Answer from the drawing. Dimensions are ordinates in mm from the lowest x, y and z of the part. A direction names the side the tool comes from. Coordinates: 2 decimals unless noted, no trailing zeros. Write each loop counter-clockwise with the first axis right and the second up, starting at its lowest first coordinate (ties: lowest second). Pieces come first, ordered by that corner, then holes.
(1) The part is cut by section B-B on z = 7.5. Determine the outline of the cut face in (x, y), plus the area to 3 significant figures.
(2) The part is cut by section D-D on x = 13.5. Determine the outline of the cut face in (y, z).
(3) The part is cut by section A-A on x = 7.5. Determine the outline of the cut face in (y, z).
(4) For a pull along Z with two mould halves and no side action, classify the marked faces 1 and 2 as +Z half, -Z half, draft (parallel to the pull), parting line (faces both ways), or undercut.
(5) Which of the six approach directions +Z, -Z, +X, -X, +Y, -Y give full straight-line access (tool end or side, diameter ignored) to the marked faces 3 and 4?
(6) Straight lines are drawn through the part: line 1 (X direction, y = 0.3, z = 7.5); line 2 (X direction, y = 2.45, z = 7.5). For each, find the intervals that lie inside material, in ascending order.
(7) The part is cut by section C-C on y = 2.35. Determine the outline of the cut face in (x, z).
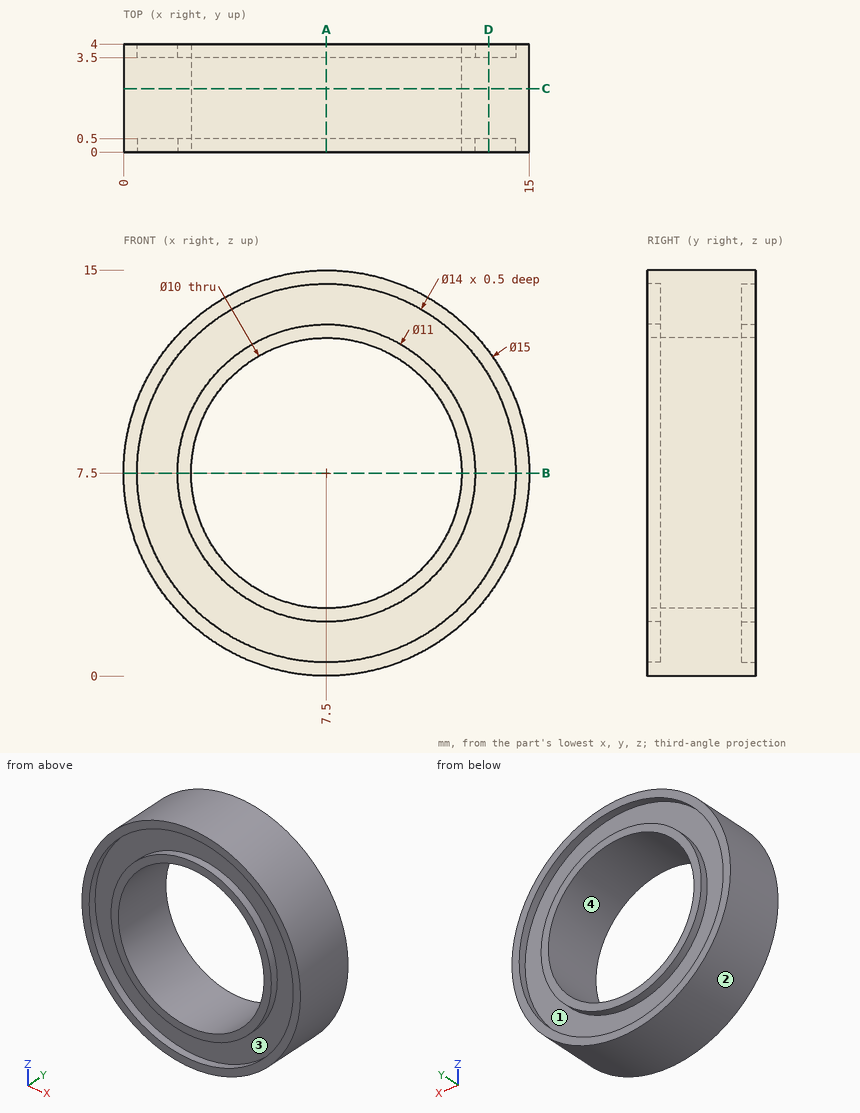
Model answer:
1. outline: (0, 0) - (0.5, 0) - (0.5, 0.5) - (2, 0.5) - (2, 0) - (2.5, 0) - (2.5, 4) - (2, 4) - (2, 3.5) - (0.5, 3.5) - (0.5, 4) - (0, 4) - close; (12.5, 0) - (13, 0) - (13, 0.5) - (14.5, 0.5) - (14.5, 0) - (15, 0) - (15, 4) - (14.5, 4) - (14.5, 3.5) - (13, 3.5) - (13, 4) - (12.5, 4) - close
1. area: 17.0 mm2
2. outline: (0, 3) - (4, 3) - (4, 3.89) - (3.5, 3.89) - (3.5, 11.11) - (4, 11.11) - (4, 12) - (0, 12) - (0, 11.11) - (0.5, 11.11) - (0.5, 3.89) - (0, 3.89) - close
3. outline: (0, 0) - (4, 0) - (4, 0.5) - (3.5, 0.5) - (3.5, 2) - (4, 2) - (4, 2.5) - (0, 2.5) - (0, 2) - (0.5, 2) - (0.5, 0.5) - (0, 0.5) - close; (0, 12.5) - (4, 12.5) - (4, 13) - (3.5, 13) - (3.5, 14.5) - (4, 14.5) - (4, 15) - (0, 15) - (0, 14.5) - (0.5, 14.5) - (0.5, 13) - (0, 13) - close
4. face 1: undercut
4. face 2: parting line
5. face 3: -Y
5. face 4: +Y, -Y
6. line 1: x = 0 to 0.5, 2 to 2.5, 12.5 to 13, 14.5 to 15
6. line 2: x = 0 to 2.5, 12.5 to 15
7. outline: circle Ø15 at (7.5, 7.5); hole circle Ø10 at (7.5, 7.5)
